For this review, take the finished solid that the model builds, in its own axes (mm). Face numbers are marked on the shaded views. A direction names the side the tool comes from. Round coordinates to 2 decimals unless told otherwise and drop trailing zeros. Order: outer loops, then holes, each group sorted by start corner. A loop starts at its lowest first (then second) coordinate and runs counter-clockwise, first axis right, second up. Notation, with made-up numbers: (61.5, 9.25) -> (89.5, 9.25) arc R24 ccw to (89.5, 27.25) -> close; hole circle Ø6 at (37, 24.25). An arc over 180 degrees is marked (long way). Put each result on its own line as item: value. Start each with the question number.
```python
from build123d import *

# Parameters (mm, degrees)
BOSS_EXTRUDE1_DEPTH = 10
FILLET1_R           = 1
FILLET2_R           = 0.5


with BuildPart() as part:
    # Sketch1 → Boss-Extrude1 (new body)
    with BuildSketch(Plane.XZ.offset(10)):
        Polygon((2.804347826, 17.533503473), (5.304347826, 19.924807821), (5.304347826, 29.324187975), (9.169667061, 31.480524519), (10.595176157, 31.480524519), (10.577761024, 29.730396695), (12.012614665, 29.730396695), (11.981340388, 33.141498149), (8.981340388, 33.141498149), (3.804347826, 30.1525601), (3.804347826, 21.359590429), (2.804347826, 21.359590429), (2.804347826, 30.924807821), (7.452279989, 33.608292706), (7.452279989, 39.375896583), (8.502279989, 39.375896583), (8.502279989, 36.050651768), (9.328366946, 36.050651768), (9.328366946, 40.650651768), (1.538219203, 40.650651768), (-0.195652174, 33.954999595), (-0.195652174, 58.52173913), (-7.269565217, 58.52173913), (-7.269565217, 55.52173913), (-6.313043478, 55.52173913), (-6.313043478, 56.52173913), (-4.713043478, 56.52173913), (-4.713043478, 55.52173913), (-2.869565217, 55.52173913), (-2.869565217, 4.387220823), (-2.869565217, -9.434782609), (-2.869565217, -30.47826087), (-4.713043478, -30.47826087), (-4.713043478, -31.47826087), (-6.313043478, -31.47826087), (-6.313043478, -30.47826087), (-7.269565217, -30.47826087), (-7.269565217, -33.47826087), (-0.195652174, -33.47826087), (-0.195652174, -6.777713361), (2.804347826, -6.777713361), (2.804347826, 2.073965174), (11.146243443, 2.073965174), (11.146243443, -21.034930407), (13.146243443, -21.034930407), (13.146243443, 3.987008652), (8.502279989, 5.232418322), (8.502279989, 4.275896583), (7.452279989, 4.275896583), (7.452279989, 5.232418322), (2.804347826, 3.987008652), align=None)
        Polygon((2.31416262, 31.796499798), (2.31416262, 39.650651768), (5.638358328, 39.650651768), (5.638358328, 33.715725085), align=None, mode=Mode.SUBTRACT)
    extrude(amount=-BOSS_EXTRUDE1_DEPTH)

    # Fillet1
    # the kernel refuses this fillet: 1 mm, written as the material it adds along each edge
    with BuildSketch(Plane(origin=(2.804347826, -10, 2.073965174), x_dir=(1, 0, 0), z_dir=(0, 1, 0)), Plane(origin=(-0.195652174, -10, -6.777713361), x_dir=(1, 0, 0), z_dir=(0, 1, 0)), Plane(origin=(11.146243443, -10, 2.073965174), x_dir=(0, 0, -1), z_dir=(0, 1, 0))) as fillet1_piece_1:
        with BuildLine():
            CenterArc((FILLET1_R, FILLET1_R), FILLET1_R, 180, 90)
            Line((0, FILLET1_R), (0, 0))
            Line((0, 0), (FILLET1_R, 0))
        make_face()
    extrude(amount=10)
    with BuildSketch(Plane(origin=(5.304347826, -10, 29.324187975), x_dir=(0.8732987298442874, 0, 0.48718510696895734), z_dir=(0, 1, 0))) as fillet1_piece_2:
        with BuildLine():
            CenterArc((FILLET1_R * 0.587215892462, FILLET1_R), FILLET1_R, 209.155734131, 60.844265869)
            Line((-FILLET1_R * 0.286082837383, FILLET1_R * 0.512814893031), (0, 0))
            Line((0, 0), (FILLET1_R * 0.587215892462, 0))
        make_face()
    extrude(amount=10)
    # the kernel refuses this fillet: 1 mm, written as the material it takes off along each edge
    with BuildSketch(Plane(origin=(11.981340388, -12.47718412, 33.141498149), x_dir=(0.009167995584995172, 0, -0.9999579730453443), z_dir=(0, 1, 0))) as fillet1_2_piece_1:
        with BuildLine():
            CenterArc((FILLET1_R * 0.990873647817, FILLET1_R), FILLET1_R, 180.525294812, 89.474705188)
            Line((-FILLET1_R * 0.00908432522847, FILLET1_R * 0.990832004415), (0, 0))
            Line((0, 0), (FILLET1_R * 0.990873647817, 0))
        make_face()
    extrude(amount=14.954368239, mode=Mode.SUBTRACT)
    with BuildSketch(Plane(origin=(10.577761024, -12.525000715, 29.730396695), x_dir=(0.009950285545768225, 0, 0.9999504946833906), z_dir=(0, 1, 0))) as fillet1_2_piece_2:
        with BuildLine():
            CenterArc((FILLET1_R * 1.01000028593, FILLET1_R), FILLET1_R, 179.429881225, 90.570118775)
            Line((FILLET1_R * 0.0100497912463, FILLET1_R * 1.00995028555), (0, 0))
            Line((0, 0), (FILLET1_R * 1.01000028593, 0))
        make_face()
    extrude(amount=15.05000143, mode=Mode.SUBTRACT)
    with BuildSketch(Plane(origin=(12.012614665, -12.523026024, 29.730396695), x_dir=(-1, 0, 0), z_dir=(0, 1, 0))) as fillet1_2_piece_3:
        with BuildLine():
            CenterArc((FILLET1_R * 1.00921040963, FILLET1_R), FILLET1_R, 179.474705188, 90.525294812)
            Line((FILLET1_R * 0.00925243657978, FILLET1_R * 1.00916799558), (0, 0))
            Line((0, 0), (FILLET1_R * 1.00921040963, 0))
        make_face()
    extrude(amount=15.046052048, mode=Mode.SUBTRACT)
    with BuildSketch(Plane(origin=(13.146243443, -12.5, -21.034930407), x_dir=(-1, 0, 0), z_dir=(0, 1, 0)), Plane(origin=(2.804347826, -12.5, -6.777713361), x_dir=(-1, 0, 0), z_dir=(0, 1, 0)), Plane(origin=(11.146243443, -12.5, -21.034930407), x_dir=(0, 0, 1), z_dir=(0, 1, 0)), Plane(origin=(-0.195652174, -12.5, -33.47826087), x_dir=(-1, 0, 0), z_dir=(0, 1, 0)), Plane(origin=(-7.269565217, -12.5, -33.47826087), x_dir=(0, 0, 1), z_dir=(0, 1, 0)), Plane(origin=(-7.269565217, -12.5, 58.52173913), x_dir=(1, 0, 0), z_dir=(0, 1, 0)), Plane(origin=(-0.195652174, -12.5, 58.52173913), x_dir=(0, 0, -1), z_dir=(0, 1, 0)), Plane(origin=(9.328366946, -12.5, 40.650651768), x_dir=(0, 0, -1), z_dir=(0, 1, 0))) as fillet1_2_piece_4:
        with BuildLine():
            CenterArc((FILLET1_R, FILLET1_R), FILLET1_R, 180, 90)
            Line((0, FILLET1_R), (0, 0))
            Line((0, 0), (FILLET1_R, 0))
        make_face()
    extrude(amount=15, mode=Mode.SUBTRACT)
    with BuildSketch(Plane(origin=(13.146243443, -11.917893225, 3.987008652), x_dir=(0, 0, -1), z_dir=(0, 1, 0))) as fillet1_2_piece_5:
        with BuildLine():
            CenterArc((FILLET1_R * 0.76715728997, FILLET1_R), FILLET1_R, 195.012240475, 74.987759525)
            Line((-FILLET1_R * 0.198713221058, FILLET1_R * 0.740974603702), (0, 0))
            Line((0, 0), (FILLET1_R * 0.76715728997, 0))
        make_face()
    extrude(amount=13.83578645, mode=Mode.SUBTRACT)
    with BuildSketch(Plane(origin=(1.538219203, -11.935074959, 40.650651768), x_dir=(1, 0, 0), z_dir=(0, 1, 0))) as fillet1_2_piece_6:
        with BuildLine():
            CenterArc((FILLET1_R * 0.774029983779, FILLET1_R), FILLET1_R, 194.518109178, 75.481890822)
            Line((-FILLET1_R * 0.19403847194, FILLET1_R * 0.749314011077), (0, 0))
            Line((0, 0), (FILLET1_R * 0.774029983779, 0))
        make_face()
    extrude(amount=13.870149919, mode=Mode.SUBTRACT)

    # Fillet2
    fillet2_edges = [part.edges().sort_by_distance(p)[0] for p in [
        (-7.269565217, -5, -30.47826087),
        (-7.269565217, -5, 55.52173913),
        (9.328366946, -5, 36.050651768),
    ]]
    fillet(fillet2_edges, radius=FILLET2_R)


solid = part.part
```
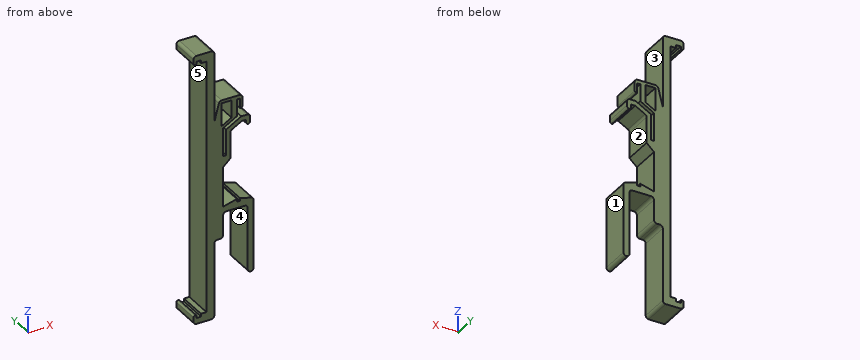
Item 1: For L1, parallel to X at y = -8, z = -9; L2, parallel to Z at x = -3.75, y = -6; L3, parallel to X at y = -5.75, z = 37, list the stretches that pass through material, from the lowest coordinate up.
Item 2: Consider section A-A, the plane x = -5.5. Write out the cut boundary in (y, z).
Item 3: Consider section C-C, the plane z = 46. Write out the cut boundary in (x, y).
Item 4: Mouldability with a two-part tool opening along Z and no side actions: class the marked faces 1 and 2 as +Z half, -Z half, draft (parallel to the pull), parting line (faces both ways), or undercut.
Item 5: Consider section B-B, the plane z = -17. Write out the cut boundary in (x, y).
Item 6: Tool access review of the marked faces 3, 4 and 5: name each direction out of +Z, -Z, +X, -X, +Y, -Y from which nothing blocks a thin tool from reaching the whole face with its end or side.
Item 7: Insertion check: pin 1 Ø1.8 at (y, z) = (-2.5, 35.5) entering from -X; pin 2 Ø1.1 at (x, y) = (3.5, -6.5) entering from +Z; pin 3 Ø3 at (x, y) = (3.5, -9) entering from -Z. Each pin has a flat end and moves straight along its axis. Give the tip position at first contact, or say it passes through.
Evaluation:
1. L1: x = -2.87 to -0.2, 11.15 to 13.15
1. L2: z = -33.48 to -30.48, 55.52 to 58.52
1. L3: x = -2.87 to -0.2, 0.59 to 2.31, 5.64 to 7.45, 8.5 to 9.33
2. outline: (-10, -33.48) -> (0, -33.48) -> (0, -31.48) -> (-10, -31.48) -> close; (-10, 56.52) -> (0, 56.52) -> (0, 58.52) -> (-10, 58.52) -> close
3. outline: (-2.87, -10) -> (-0.2, -10) -> (-0.2, 0) -> (-2.87, 0) -> close
4. face 1: draft
4. face 2: undercut
5. outline: (-2.87, -10) -> (-0.2, -10) -> (-0.2, 0) -> (-2.87, 0) -> close; (11.15, -10) -> (13.15, -10) -> (13.15, 0) -> (11.15, 0) -> close
6. face 3: +Z, +Y, -Y
6. face 4: -Z, +Y, -Y
6. face 5: -X, +Y, -Y
7. pin 1: stops at x = -2.87
7. pin 2: stops at z = 40.65
7. pin 3: stops at z = -6.76
